from build123d import *

# Parameters (mm, degrees)
SKETCH2_R          = 5
CUT_EXTRUDE1_DEPTH = 27


with BuildPart() as part:
    # Sketch1 → Revolve1 (revolve)
    with BuildSketch(Plane(origin=(0, 0, 0), x_dir=(0, 0, -1), z_dir=(1, 0, 0))):
        Polygon((-17.5, 48), (17.5, 48), (17.5, 38), (5.5, 35), (-5.5, 35), (-17.5, 38), align=None)
        Polygon((-5.5, 18), (-5.5, 10), (5.5, 10), (5.5, 18), (5.5, 35), (-5.5, 35), align=None)
        Polygon((5.5, 18), (5.5, 10), (20.5, 10), (20.5, 16), align=None)
        Polygon((-20.5, 16), (-20.5, 10), (-5.5, 10), (-5.5, 18), align=None)
    revolve(axis=Axis((0, 0, 20.5), (0, 0, -1)))

    # Sketch2 → Cut-Extrude1 (cut, through all)
    with BuildSketch(Plane(origin=(0, 0, -5.5), x_dir=(-1, 0, 0), z_dir=(0, 0, -1))):
        with Locations((0, 26.5)):
            Circle(SKETCH2_R)
        with Locations((26.5, 0)):
            Circle(SKETCH2_R)
        with Locations((0, -26.5)):
            Circle(SKETCH2_R)
        with Locations((-26.5, 0)):
            Circle(SKETCH2_R)
    extrude(amount=-CUT_EXTRUDE1_DEPTH, mode=Mode.SUBTRACT)


solid = part.part
Can you work these out from the model? Positions are in its coordinate system, mm. A direction names the side the tool comes from. Coordinates: 2 decimals unless noted, no trailing zeros. Order: outer loops, then holes, each group sorted by start corner. A loop starts at its lowest first (then second) coordinate and runs counter-clockwise, first axis right, second up. Notation, with made-up numbers: M 29.25,73.5 L 76.25,73.5 A19 ccw 76.25,88.5 Z; hole C -28,-9.5 d5. An arc over 180 degrees is marked long. Write item = value, one per line.
(1) For pin 1 Ø16 at (x, y) = (0, 26.5) entering from -Z; pin 2 Ø1.5 at (y, z) = (24.5, -2.5) entering from -X; pin 3 Ø3 at (x, y) = (-28, -30.5) entering from +Z, each with a flat end and sliding along its axis, tell me the tip position at first contact or that it passes through.
Results are:
pin_1 = -5.5
pin_2 = -41.71
pin_3 = 17.5
(2) I need wall thicknesses on line 1 along X through (y, z) = (-10.5, -15.5); line 2 along Z through (x, y) = (22.5, -19); line 3 along Y through (x, z) = (19, 11.5). Which ranges of each line are inside material? Lowest first, please. Write a range as [from, to].
Results are:
line_1 = [-46.84, -36], [-12.94, 12.94], [36, 46.84]
line_2 = [-5.5, 5.5]
line_3 = [-44.08, -31.16], [31.16, 44.08]
(3) Suppose I cut it at C-C on y = -3.5. State how many separate pieces and enclosed holes the cut face has, plus the area to 3 significant figures.
Results are:
separate_pieces = 4
enclosed_holes = 0
area = 1,680 mm2
(4) Suppose I cut it at B-B on z = 11.5. Please give me the cut outline in (x, y), plus the area to 3 significant figures.
Results are:
outline = C 0,0 d96; C 0,0 d34.4; hole C 0,0 d73; hole C 0,0 d20
area = 3,670 mm2
(5) Suppose I cut it at A-A on z = 1.5. Please give me the cut outline in (x, y).
Results are:
outline = C 0,0 d96; hole C -26.5,0 d10; hole C 0,0 d20; hole C 0,-26.5 d10; hole C 0,26.5 d10; hole C 26.5,0 d10
(6) For faces 1 (the face through (-15, -15, -5.5)), 2 (the face through (-15, 15, 5.5)), 3 (the face through (2.11, -47.954, -0.245)), which set-ups out of +Z, -Z, +X, -X, +Y, -Y let a thin tool reach every point of the face, with its end or its side?
Results are:
face_1 = -Z
face_2 = +Z
face_3 = +Z, -Z
